Check sheet for the modelled part. Datum: model origin and axes. Units: mm. Give positions to 0.01 mm unless a question says otherwise; leave off trailing zeros. Order: outer loops, then holes, each group sorted by start corner. A loop starts at its lowest first (then second) coordinate and runs counter-clockwise, first axis right, second up.
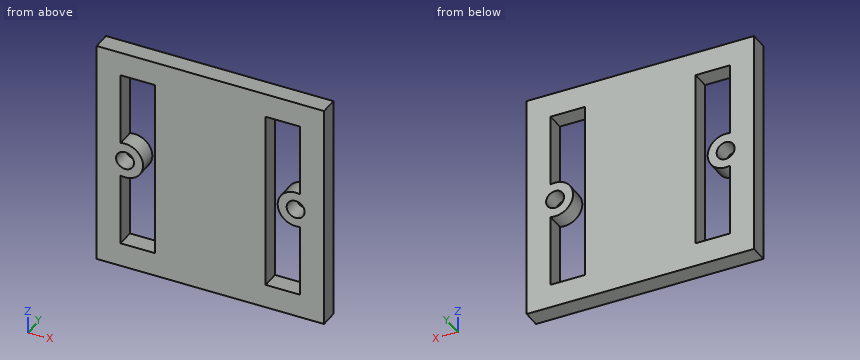
```python
from build123d import *

# Parameters (mm, degrees)
SKETCH1_W           = 38
SKETCH1_H           = 38
SKETCH1_R           = 1.5
BOSS_EXTRUDE1_DEPTH = 3


with BuildPart() as part:
    # Sketch1 → Boss-Extrude1 (new body)
    with BuildSketch(Plane(origin=(0, 0, 0), x_dir=(1, 0, 0), z_dir=(0, 1, 0))):
        Rectangle(SKETCH1_W, SKETCH1_H)
        with BuildLine():
            ThreePointArc((-15, -2.90473751), (-11.25, 0), (-15, 2.90473751))
            Line((-15, 2.90473751), (-15, 15))
            Line((-15, 15), (-9.25, 15))
            Line((-9.25, 15), (-9.25, -15))
            Line((-9.25, -15), (-15, -15))
            Line((-15, -15), (-15, -2.90473751))
        make_face(mode=Mode.SUBTRACT)
        with Locations(Location((-14.25, 0, 0), (0, 0, 270))):
            Circle(SKETCH1_R, mode=Mode.SUBTRACT)
        with BuildLine():
            Line((15, -15), (9.25, -15))
            Line((9.25, -15), (9.25, 15))
            Line((9.25, 15), (15, 15))
            Line((15, 15), (15, 2.90473751))
            ThreePointArc((15, 2.90473751), (11.25, 0), (15, -2.90473751))
            Line((15, -2.90473751), (15, -15))
        make_face(mode=Mode.SUBTRACT)
        with Locations(Location((14.25, 0, 0), (0, 0, 270))):
            Circle(SKETCH1_R, mode=Mode.SUBTRACT)
    extrude(amount=BOSS_EXTRUDE1_DEPTH)


solid = part.part
```
(1) Cross-section at B-B on x = 14.25. Enter the section's corners in (y, z), then the cut area to 3 significant figures.
Response values:
outline: (0, -19) - (3, -19) - (3, -15) - (0, -15) - close; (0, -3) - (3, -3) - (3, -1.5) - (0, -1.5) - close; (0, 1.5) - (3, 1.5) - (3, 3) - (0, 3) - close; (0, 15) - (3, 15) - (3, 19) - (0, 19) - close
area: 33.0 mm2
(2) Cross-section at C-C on y = 1. Enter the section's corners in (x, z).
Response values:
outline: (-19, -19) - (19, -19) - (19, 19) - (-19, 19) - close; hole circle Ø3 at (-14.25, 0); hole (-15, -15) - (-9.25, -15) - (-9.25, 15) - (-15, 15) - (-15, 2.9) arc R3 cw (long way) to (-15, -2.9) - close; hole (9.25, -15) - (15, -15) - (15, -2.9) arc R3 cw (long way) to (15, 2.9) - (15, 15) - (9.25, 15) - close; hole circle Ø3 at (14.25, 0)
(3) Gauge pin test, flat end, axial feed: pin 1 Ø2.5 at (x, z) = (-14.25, 0) entering from +Y. Record the tip position at first contact, or that the pin passes through.
Response values:
pin 1: passes through
(4) Cross-section at D-D on z = 0. Enter the section's corners in (x, y), then the cut area to 3 significant figures.
Response values:
outline: (-19, 0) - (-15.75, 0) - (-15.75, 3) - (-19, 3) - close; (-12.75, 0) - (-11.25, 0) - (-11.25, 3) - (-12.75, 3) - close; (-9.25, 0) - (9.25, 0) - (9.25, 3) - (-9.25, 3) - close; (11.25, 0) - (12.75, 0) - (12.75, 3) - (11.25, 3) - close; (15.75, 0) - (19, 0) - (19, 3) - (15.75, 3) - close
area: 84.0 mm2
(5) Cross-section at A-A on z = 13. Enter the section's corners in (x, y), then the cut area to 3 significant figures.
Response values:
outline: (-19, 0) - (-15, 0) - (-15, 3) - (-19, 3) - close; (-9.25, 0) - (9.25, 0) - (9.25, 3) - (-9.25, 3) - close; (15, 0) - (19, 0) - (19, 3) - (15, 3) - close
area: 79.5 mm2
(6) Material ranges on L1, parallel to X at y = 2.8, z = 9.5; L2, parallel to X at y = 1.8, z = 1; L3, parallel to Z at x = -14, y = 1.15, recorded low to high.
Response values:
L1: x = -19 to -15, -9.25 to 9.25, 15 to 19
L2: x = -19 to -15.37, -13.13 to -11.42, -9.25 to 9.25, 11.42 to 13.13, 15.37 to 19
L3: z = -19 to -15, -2.99 to -1.48, 1.48 to 2.99, 15 to 19
